Geometry: final body of the model. Coordinates: model frame, mm. A direction names the side the tool comes from. Coordinates: 2 decimals unless noted, no trailing zeros. Loops run counter-clockwise (first coordinate to the right, second up) from the corner with the lowest first, then second, coordinate; pieces in that order, holes last. Notation, with made-up numbers: M 83.25,81.25 L 133.25,81.25 A4 ccw 133.25,85.25 Z; hole C 19,39.25 d5. An arc over 180 degrees is marked long. Write item = value, one per line. Start each with the question number.
```python
from build123d import *

# Parameters (mm, degrees)
EXTRUDE_1_DEPTH     = 11.3
CUT_EXTRUDE_1_DEPTH = 4.6
SKETCH_3_W          = 63.8
SKETCH_3_H          = 30.3
CUT_EXTRUDE_2_DEPTH = 4.7
SKETCH_4_W          = 4.2
SKETCH_4_H          = 0.7
CUT_EXTRUDE_3_DEPTH = 0.5
SKETCH_5_W          = 4.2
SKETCH_5_H          = 0.7
CUT_EXTRUDE_4_DEPTH = 0.5
FILLET_4_R          = 0.8


with BuildPart() as part:
    # 草图1 → 凸台-拉伸1 (new body)
    with BuildSketch(Plane(origin=(0, 0, 0), x_dir=(1, 0, 0), z_dir=(0, 1, 0))):
        with BuildLine():
            Line((-32.2, 17.15), (32.2, 17.15))
            ThreePointArc((32.2, 17.15), (33.402081528, 16.652081528), (33.9, 15.45))
            Line((33.9, 15.45), (33.9, -15.45))
            ThreePointArc((33.9, -15.45), (33.402081528, -16.652081528), (32.2, -17.15))
            Line((32.2, -17.15), (-32.2, -17.15))
            ThreePointArc((-32.2, -17.15), (-33.402081528, -16.652081528), (-33.9, -15.45))
            Line((-33.9, -15.45), (-33.9, 15.45))
            ThreePointArc((-33.9, 15.45), (-33.402081528, 16.652081528), (-32.2, 17.15))
        make_face()
    extrude(amount=EXTRUDE_1_DEPTH)

    # 草图2 → 切除-拉伸1 (cut)
    with BuildSketch(Plane(origin=(0, 11.3, 0), x_dir=(1, 0, 0), z_dir=(0, 1, 0))):
        with BuildLine():
            Line((32.9, -15.45), (32.9, 15.45))
            ThreePointArc((32.9, 15.45), (32.694974747, 15.944974747), (32.2, 16.15))
            Line((32.2, 16.15), (-32.2, 16.15))
            ThreePointArc((-32.2, 16.15), (-32.694974747, 15.944974747), (-32.9, 15.45))
            Line((-32.9, 15.45), (-32.9, -15.45))
            ThreePointArc((-32.9, -15.45), (-32.694974747, -15.944974747), (-32.2, -16.15))
            Line((-32.2, -16.15), (32.2, -16.15))
            ThreePointArc((32.2, -16.15), (32.694974747, -15.944974747), (32.9, -15.45))
        make_face()
    extrude(amount=-CUT_EXTRUDE_1_DEPTH, mode=Mode.SUBTRACT)

    # 草图3 → 切除-拉伸2 (cut)
    with BuildSketch(Plane(origin=(0, 6.7, 0), x_dir=(1, 0, 0), z_dir=(0, 1, 0))):
        Rectangle(SKETCH_3_W, SKETCH_3_H)
    extrude(amount=-CUT_EXTRUDE_2_DEPTH, mode=Mode.SUBTRACT)

    # 草图4 → 切除-拉伸3 (cut)
    with BuildSketch(Plane(origin=(-32.9, 0, 0), x_dir=(0, 0, -1), z_dir=(1, 0, 0))):
        with Locations((0, 8.82)):
            Rectangle(SKETCH_4_W, SKETCH_4_H)
    cut_extrude_3 = extrude(amount=-CUT_EXTRUDE_3_DEPTH, mode=Mode.SUBTRACT)

    # 镜向1: 切除-拉伸3 across plane
    add(cut_extrude_3.mirror(Plane(origin=(0, 0, 0), x_dir=(0, 0, 1), z_dir=(1, 0, 0))), mode=Mode.SUBTRACT)

    # 草图5 → 切除-拉伸4 (cut)
    with BuildSketch(Plane(origin=(0, 0, 16.15), x_dir=(-1, 0, 0), z_dir=(0, 0, -1))):
        with Locations((-24.8, 8.82)):
            Rectangle(SKETCH_5_W, SKETCH_5_H)
        with Locations((24.8, 8.82)):
            Rectangle(SKETCH_5_W, SKETCH_5_H)
    cut_extrude_4 = extrude(amount=-CUT_EXTRUDE_4_DEPTH, mode=Mode.SUBTRACT)

    # 镜向2: 切除-拉伸4 across plane
    add(cut_extrude_4.mirror(Plane.XY), mode=Mode.SUBTRACT)

    # 圆角4
    fillet_4_edges = [part.edges().sort_by_distance(p)[0] for p in [
        (-33.402081528, 11.3, -16.652081528),
        (-33.9, 11.3, 0),
        (-33.402081528, 11.3, 16.652081528),
        (0, 11.3, 17.15),
        (33.402081528, 11.3, 16.652081528),
        (33.9, 11.3, 0),
        (33.402081528, 11.3, -16.652081528),
        (0, 11.3, -17.15),
    ]]
    fillet(fillet_4_edges, radius=FILLET_4_R)


solid = part.part
```
Item 1: Section query A-A (z = -14). Return the cut outline in (x, y).
Item 2: Pull-direction query (Z, two-part tool) for faces 3 (the flat face through (-32.9, 10, 0)), 4 (the flat face through (0, 5, 17.15)), 5 (the flat face through (0, 5, -17.15)), 6 (the flat face through (-33.9, 5, 0)); classes: released by +Z, released by -Z, zero draft, split by the parting line, or undercut.
Item 3: Section query B-B (y = 3.25). Return the cut outline in (x, z), plus the area to 3 significant figures.
Item 4: Section query D-D (x = 24.5). Return the cut outline in (y, z), plus the area to 3 significant figures.
Item 5: Section query C-C (x = 10). Return the cut outline in (y, z).
Item 6: Line query: line 1 (X direction, y = 2.25, z = -3); line 2 (Z direction, x = -29, y = 6.5); line 3 (X direction, y = 9, z = 11). Output: solid intervals per line, ascending. Write a range as from..to.
Item 7: First-contact query: pin 1 (5 mm diameter, centred on x = 24.5, z = -11, fed in from +Y). Flat tip, straight axial feed; report the tip coordinate or a pass-through.
Item 8: Reachability of faces 1 (the flat face through (0, 2, 0)), 2 (the cylindrical face through (33.389, 5.176, -16.665)) from +Z, -Z, +X, -X, +Y, -Y: full face, straight path, thin tool, end or side. Return the list, or none.
Verdict:
q1.outline = M -33.9,0 L 33.9,0 L 33.9,10.5 A0.8 ccw 33.1,11.3 L 32.9,11.3 L 32.9,6.7 L 31.9,6.7 L 31.9,2 L -31.9,2 L -31.9,6.7 L -32.9,6.7 L -32.9,11.3 L -33.1,11.3 A0.8 ccw -33.9,10.5 Z
q2.face_3 = undercut
q2.face_4 = released by +Z
q2.face_5 = released by -Z
q2.face_6 = zero draft
q3.outline = M -33.9,-15.45 A1.7 ccw -32.2,-17.15 L 32.2,-17.15 A1.7 ccw 33.9,-15.45 L 33.9,15.45 A1.7 ccw 32.2,17.15 L -32.2,17.15 A1.7 ccw -33.9,15.45 Z; hole M -31.9,-15.15 L 31.9,-15.15 L 31.9,15.15 L -31.9,15.15 Z
q3.area = 390 mm2
q4.outline = M 0,-17.15 L 10.5,-17.15 A0.8 ccw 11.3,-16.35 L 11.3,-16.15 L 9.17,-16.15 L 9.17,-16.65 L 8.47,-16.65 L 8.47,-16.15 L 6.7,-16.15 L 6.7,-15.15 L 2,-15.15 L 2,15.15 L 6.7,15.15 L 6.7,16.15 L 8.47,16.15 L 8.47,16.65 L 9.17,16.65 L 9.17,16.15 L 11.3,16.15 L 11.3,16.35 A0.8 ccw 10.5,17.15 L 0,17.15 Z
q4.area = 95.6 mm2
q5.outline = M 0,-17.15 L 10.5,-17.15 A0.8 ccw 11.3,-16.35 L 11.3,-16.15 L 6.7,-16.15 L 6.7,-15.15 L 2,-15.15 L 2,15.15 L 6.7,15.15 L 6.7,16.15 L 11.3,16.15 L 11.3,16.35 A0.8 ccw 10.5,17.15 L 0,17.15 Z
q6.line_1 = -33.9..-31.9, 31.9..33.9
q6.line_2 = -17.15..-15.15, 15.15..17.15
q6.line_3 = -33.9..-32.9, 32.9..33.9
q7.pin_1 = 2
q8.face_1 = +Y
q8.face_2 = -Z, +X, +Y, -Y
